For this review, use the dimensioned drawing (mm, ordinates from the lowest corner) and the shaded views. A direction names the side the tool comes from. Give positions to 0.01 mm unless a question says otherwise; leave off trailing zeros. Loops run counter-clockwise (first coordinate to the right, second up) from the corner with the lowest first, then second, coordinate; pieces in that order, holes last. Notation, with made-up numbers: (80, -20.5) - (95, -20.5) arc R14 ccw to (95, 2.5) - close; hole circle Ø4 at (-28.5, 10.25). An arc over 180 degrees is marked (long way). Write each question's results on one line, items separated by ' | '.
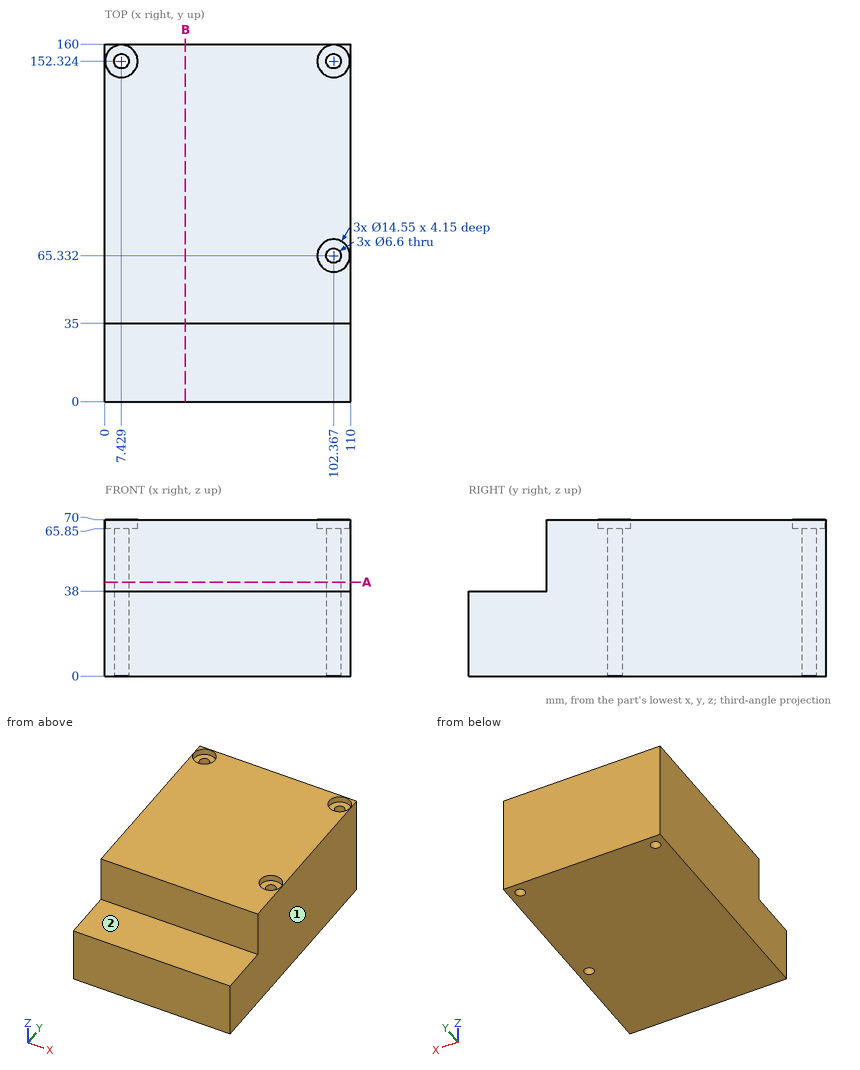
Item 1: We need section A-A on z = 42. Give the boundary of the cut face in (x, y).
Output values:
outline: (0, 35) - (110, 35) - (110, 160) - (0, 160) - close; hole circle Ø6.6 at (7.43, 152.32); hole circle Ø6.6 at (102.37, 65.33); hole circle Ø6.6 at (102.37, 152.32)
Item 2: Tool access review of the marked faces 1 and 2: name each direction out of +Z, -Z, +X, -X, +Y, -Y from which nothing blocks a thin tool from reaching the whole face with its end or side.
Output values:
face 1: +Z, -Z, +X, +Y, -Y | face 2: +Z, +X, -X, -Y
Item 3: Wall thickness on probe 1 along Y at (x, z) = (102.5, 19.5) (1 decimal); probe 2 along Z at (x, y) = (101, 24); probe 3 along Y at (x, z) = (22, 40): over which ranges is each line inside the solid? List them lowest first.
Output values:
probe 1: y = 0 to 62, 68.6 to 149, 155.6 to 160 | probe 2: z = 0 to 38 | probe 3: y = 35 to 160
Item 4: Clearance check with flat-ended pins moving along their axes: P1, Ø5.5, axis at x = 7.43, y = 152.32, coming from the -Z side; P2, Ø3, axis at x = 57, z = 58, coming from the -Y side; P3, Ø17.5, axis at x = 71.5, y = 17.5, coming from the +Z side; P4, Ø7.5, axis at x = 99.5, y = 150.5, coming from the +Z side. State where each tip first meets the part, or that it passes through.
Output values:
P1: passes through | P2: stops at y = 35 | P3: stops at z = 38 | P4: stops at z = 65.85
Item 5: We need section B-B on x = 36. Give the boundary of the cut face in (y, z), then the cut area to 3 significant figures.
Output values:
outline: (0, 0) - (160, 0) - (160, 70) - (35, 70) - (35, 38) - (0, 38) - close | area: 10,100 mm²
